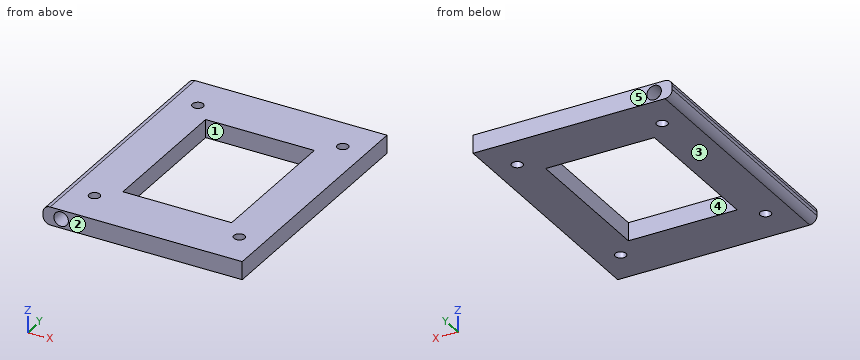
```python
from build123d import *

# Parameters (mm, degrees)
SKETCH1_W           = 70
SKETCH1_H           = 55
BOSS_EXTRUDE1_DEPTH = 5
SKETCH2_R           = 2
CUT_EXTRUDE1_DEPTH  = 4.5
SKETCH3_R           = 2
CUT_EXTRUDE2_DEPTH  = 4.5
FILLET1_R           = 2
SKETCH4_R           = 1.5
SKETCH4_W           = 30
SKETCH4_H           = 40
CUT_EXTRUDE3_DEPTH  = 6


with BuildPart() as part:
    # Sketch1 → Boss-Extrude1 (new body)
    with BuildSketch(Plane(origin=(0, 0, 0), x_dir=(0, 1, 0), z_dir=(0, 0, 1))):
        with Locations((35, 27.5)):
            Rectangle(SKETCH1_W, SKETCH1_H)
    extrude(amount=BOSS_EXTRUDE1_DEPTH)

    # Sketch2 → Cut-Extrude1 (cut)
    with BuildSketch(Plane(origin=(0, 70, 0), x_dir=(-1, 0, 0), z_dir=(0, 1, 0))):
        with Locations((50, 2.5)):
            Circle(SKETCH2_R)
    extrude(amount=-CUT_EXTRUDE1_DEPTH, mode=Mode.SUBTRACT)

    # Sketch3 → Cut-Extrude2 (cut)
    with BuildSketch(Plane.XZ):
        with Locations((-50, 2.5)):
            Circle(SKETCH3_R)
    extrude(amount=-CUT_EXTRUDE2_DEPTH, mode=Mode.SUBTRACT)

    # Fillet1
    fillet1_edges = [part.edges().sort_by_distance(p)[0] for p in [
        (-55, 35, 5),
        (-55, 35, 0),
    ]]
    fillet(fillet1_edges, radius=FILLET1_R)

    # Sketch4 → Cut-Extrude3 (cut, through all)
    with BuildSketch(Plane.XY.offset(5)):
        with Locations((-6.5, 60)):
            Circle(SKETCH4_R)
        with Locations((-46.5, 60)):
            Circle(SKETCH4_R)
        with Locations((-6.5, 10)):
            Circle(SKETCH4_R)
        with Locations((-46.5, 10)):
            Circle(SKETCH4_R)
        with Locations((-26.5, 35)):
            Rectangle(SKETCH4_W, SKETCH4_H)
    extrude(amount=-CUT_EXTRUDE3_DEPTH, mode=Mode.SUBTRACT)


solid = part.part
```
Source: CAD feature listing. Evaluate the final solid. Frame: model axes, mm. Face numbers are marked on the shaded views. A direction names the side the tool comes from. Round coordinates to 2 decimals unless told otherwise and drop trailing zeros. Write each loop counter-clockwise with the first axis right and the second up, starting at its lowest first coordinate (ties: lowest second). Pieces come first, ordered by that corner, then holes. Notation, with made-up numbers: M 15,-3 L 22,-3 A8 ccw 22,6 Z; hole C -37.75,54.5 d4. An arc over 180 degrees is marked long. Answer as a JSON object with one key per item and string values. Group by question number.
(1) First-contact query: pin 1 (5 mm diameter, centred on x = -46.5, y = 60, fed in from +Z); pin 2 (2.5 mm diameter, centred on x = -50, z = 2.5, fed in from +Y); pin 3 (2 mm diameter, centred on x = -50.5, z = 2.5, fed in from -Y). Flat tips, straight axial feed; report the tip coordinate or a pass-through.
(2) Section query B-B on y = 16.5. Output: boundary loops of the cut face in (x, z).
(3) Section query C-C on x = -6.5. Output: boundary loops of the cut face in (y, z), then the cut area to 3 significant figures.
(4) Mould query, pull axis Y, two halves, no side actions, for the marked faces 3, 4 and 5. Classes: +Y half, -Y half, draft (parallel to the pull), parting line (faces both ways), or undercut.
(5) Ray query, line 1 (Y direction, x = -6.5, z = 3.4); line 2 (X direction, y = 45.5, z = 2.75); line 3 (Y direction, x = -18.5, z = 4.45). Return the intervals inside material, ascending. Write a range as [from, to].
(6) Section query A-A on x = -27.5. Output: boundary loops of the cut face in (y, z).
(7) Section query D-D on x = -50. Output: boundary loops of the cut face in (y, z), then the cut area to 3 significant figures.
(8) Reachability of the marked faces 1 and 2 from +Z, -Z, +X, -X, +Y, -Y: full face, straight path, thin tool, end or side. Return the list, or none.
Computed values:
{
 "1": {"pin 1": "z = 5", "pin 2": "y = 65.5", "pin 3": "y = 4.5"},
 "2": {"outline": "M -55,2 A2 ccw -53,0 L -41.5,0 L -41.5,5 L -53,5 A2 ccw -55,3 Z; M -11.5,0 L 0,0 L 0,5 L -11.5,5 Z"},
 "3": {"outline": "M 0,0 L 8.5,0 L 8.5,5 L 0,5 Z; M 11.5,0 L 58.5,0 L 58.5,5 L 11.5,5 Z; M 61.5,0 L 70,0 L 70,5 L 61.5,5 Z", "area": "320 mm^2"},
 "4": {"face 3": "draft", "face 4": "undercut", "face 5": "+Y half"},
 "5": {"line 1": "[0, 8.5], [11.5, 58.5], [61.5, 70]", "line 2": "[-55, -41.5], [-11.5, 0]", "line 3": "[0, 15], [55, 70]"},
 "6": {"outline": "M 0,0 L 15,0 L 15,5 L 0,5 Z; M 55,0 L 70,0 L 70,5 L 55,5 Z"},
 "7": {"outline": "M 0,0 L 70,0 L 70,0.5 L 65.5,0.5 L 65.5,4.5 L 70,4.5 L 70,5 L 0,5 L 0,4.5 L 4.5,4.5 L 4.5,0.5 L 0,0.5 Z", "area": "314 mm^2"},
 "8": {"face 1": "+Z, -Z", "face 2": "+Z, -Z, +X, -X, -Y"}
}
